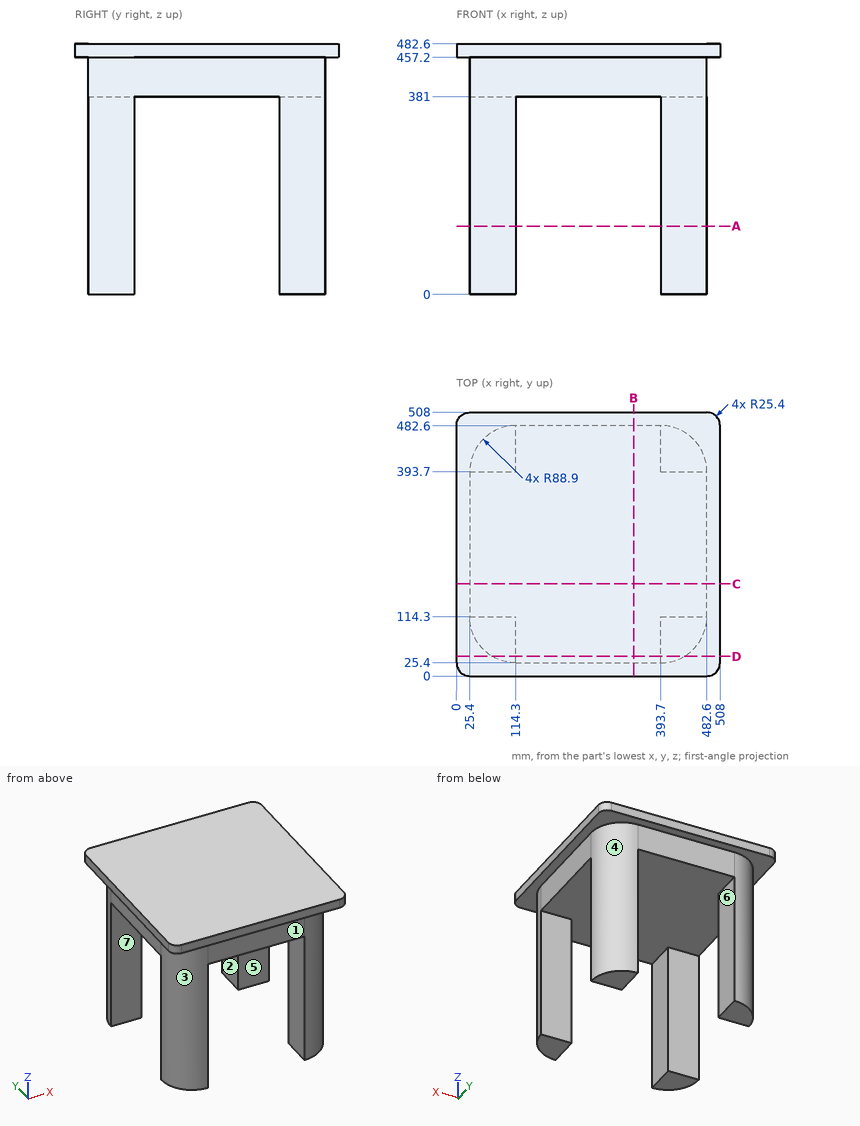
Check sheet for the drawn part. Datum: minimum x, y, z corner. Units: mm. A direction names the side the tool comes from. Coordinates: 2 decimals unless noted, no trailing zeros. Loops run counter-clockwise (first coordinate to the right, second up) from the corner with the lowest first, then second, coordinate; pieces in that order, holes last. Notation, with made-up numbers: (23, 6.25) - (61, 6.25) arc R15 cw to (61, 22.25) - close; hole circle Ø1 at (88.5, 72.5). An arc over 180 degrees is marked (long way). Put each result on its own line as item: value.
Item 1: Section check D-D (y = 38). Enter the section's corners in (x, z).
Conclusion:
outline: (0, 457.2) - (68.68, 457.2) - (68.68, 0) - (114.3, 0) - (114.3, 381) - (393.7, 381) - (393.7, 0) - (439.32, 0) - (439.32, 457.2) - (508, 457.2) - (508, 482.6) - (0, 482.6) - close
Item 2: Draft check along Y on the marked faces 4, 5, 6 and 7. Enter one of: pulls with the +Y half, pulls with the -Y half, needs draft (parallel to the pull), parting line crosses it, or undercut.
Conclusion:
face 4: pulls with the +Y half
face 5: undercut
face 6: needs draft
face 7: undercut
Item 3: Gauge pin test, flat ends, axial feed: pin 1 Ø12 at (x, z) = (364.5, 382.5) entering from +Y; pin 2 Ø8 at (x, y) = (414, 382) entering from -Z; pin 3 Ø5 at (y, z) = (71.5, 408.5) entering from -X. Record the tip position at first contact, or that the pin passes through.
Conclusion:
pin 1: stops at y = 482.6
pin 2: stops at z = 381
pin 3: stops at x = 35.06
Item 4: Scan lines: line 1 along X through (y, z) = (110.5, 352.5); line 2 along Z through (x, y) = (164, 83.5); line 3 along X through (y, z) = (412, 198). Record each from-to range of solid material in increasing order.
Conclusion:
line 1: x = 25.48 to 114.3, 393.7 to 482.52
line 2: z = 381 to 482.6
line 3: x = 27.3 to 114.3, 393.7 to 480.7
Item 5: Section check A-A (z = 131.5). Give the number of separate pieces and of enclosed holes in the cut face, then the cut area to 3 significant figures.
Conclusion:
separate pieces: 4
enclosed holes: 0
area: 24,800 mm2
Item 6: Set-up check for the marked faces 1, 2 and 3: record each of +Z, -Z, +X, -X, +Y, -Y from which the full face is reachable in a straight line by a thin tool's end or side.
Conclusion:
face 1: -Z, +X, -X, -Y
face 2: -Z, +Y, -Y
face 3: -Z, -X, -Y
Item 7: Section check B-B (x = 341.5). Enter the section's corners in (y, z), then the cut area to 3 significant figures.
Conclusion:
outline: (0, 457.2) - (25.4, 457.2) - (25.4, 381) - (482.6, 381) - (482.6, 457.2) - (508, 457.2) - (508, 482.6) - (0, 482.6) - close
area: 47,700 mm2
